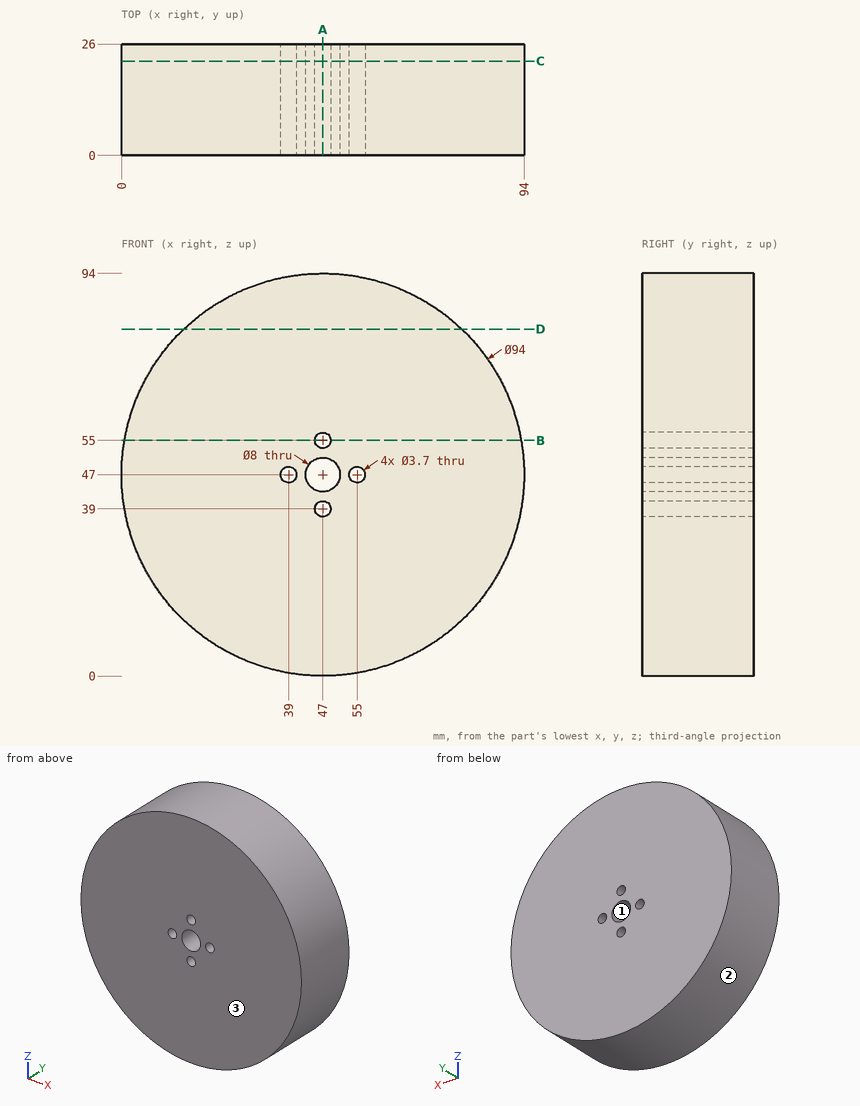
Could you check a few things on this drawing? It's one solid part, dimensions in mm from its lowest x, y, z. Coordinates: 2 decimals unless noted, no trailing zeros. Order: outer loops, then holes, each group sorted by start corner. A loop starts at its lowest first (then second) coordinate and runs counter-clockwise, first axis right, second up. Notation, with made-up numbers: (44.25, 29.5) - (68.25, 29.5) arc R22 cw to (68.25, 54.5) - close; hole circle Ø5 at (70, 71). An arc over 180 degrees is marked (long way). One line per question, with ' | ' between items.
(1) Suppose I cut it at D-D on z = 81. List the corners of the cut face in (x, y) for me.
Report:
outline: (14.55, 0) - (79.45, 0) - (79.45, 26) - (14.55, 26) - close
(2) Suppose I cut it at A-A on x = 47. List the corners of the cut face in (y, z) for me, and give its area (3 significant figures).
Report:
outline: (0, 0) - (26, 0) - (26, 37.15) - (0, 37.15) - close; (0, 40.85) - (26, 40.85) - (26, 43) - (0, 43) - close; (0, 51) - (26, 51) - (26, 53.15) - (0, 53.15) - close; (0, 56.85) - (26, 56.85) - (26, 94) - (0, 94) - close | area: 2,040 mm2
(3) If I drill on L1, parallel to Z at x = 47, y = 14.75; L2, parallel to X at y = 12, z = 45.5; L3, parallel to X at y = 21.75, z = 44, over which ranges is the centre line in solid material (lowest first)?
Report:
L1: z = 0 to 37.15, 40.85 to 43, 51 to 53.15, 56.85 to 94 | L2: x = 0.02 to 37.92, 40.08 to 43.29, 50.71 to 53.92, 56.08 to 93.98 | L3: x = 0.1 to 44.35, 49.65 to 93.9
(4) Suppose I cut it at B-B on z = 55. List the corners of the cut face in (x, y) for me.
Report:
outline: (0.69, 0) - (45.15, 0) - (45.15, 26) - (0.69, 26) - close; (48.85, 0) - (93.31, 0) - (93.31, 26) - (48.85, 26) - close
(5) Suppose I cut it at C-C on y = 22. List the corners of the cut face in (x, z) for me, and give its area (3 significant figures).
Report:
outline: circle Ø94 at (47, 47); hole circle Ø3.7 at (39, 47); hole circle Ø8 at (47, 47); hole circle Ø3.7 at (47, 39); hole circle Ø3.7 at (47, 55); hole circle Ø3.7 at (55, 47) | area: 6,850 mm2
(6) Will these pins go through, and if not, where does the flat tip stop? pin 1 (5 mm diameter, centred on x = 54, y = 11.5, fed in from +Z); pin 2 (2 mm diameter, centred on x = 47, z = 39, fed in from -Y); pin 3 (10 mm diameter, centred on y = 12.5, z = 25.5, fed in from -X); pin 4 (8 mm diameter, centred on x = 63, z = 61.5, fed in from -Y).
Report:
pin 1: stops at z = 93.78 | pin 2: passes through | pin 3: stops at x = 2.99 | pin 4: stops at y = 0
(7) If we mould it in two halves opening along Z, with no side actions, what happens to the marked faces 1, 2 and 3? For each: pulls with the +Z half, pulls with the -Z half, needs draft (parallel to the pull), parting line crosses it, or undercut.
Report:
face 1: undercut | face 2: parting line crosses it | face 3: needs draft
